```python
from build123d import *

# Parameters (mm, degrees)
BASE_FLANGE1_DEPTH       = 2.286
EDGE_FLANGE17_DEPTH      = 540.189115874
EDGE_FLANGE17_BEND_DEPTH = 539.451478538
EDGE_FLANGE18_DEPTH      = 357.000345524
EDGE_FLANGE18_BEND_DEPTH = 356.321109034
SKETCH197_R              = 12.065
CUT_EXTRUDE1_DEPTH       = 652.69497057


# Sheet-metal steps are written as plain solids
with BuildPart() as part:
    # Sketch1 → Base-Flange1 (new body)
    with BuildSketch(Plane(origin=(0, 0, 0), x_dir=(1, 0, 0), z_dir=(0, 1, 0))):
        Polygon((539.451478538, 356.320345524), (0, 356.320345524), (-0.737637336, 356.320345524), (0, 0), (539.451478538, 0), align=None)
    extrude(amount=-BASE_FLANGE1_DEPTH)

    # Edge-Flange17 section (across the edge) → Edge-Flange17 (add)
    with BuildSketch(Plane(origin=(-0.737637336, -2.286, -357.396945524), x_dir=(0, 0, 1), z_dir=(1, 0, 0))):
        with BuildLine():
            Line((-2.286, 0.7366), (-2.286, 16.15))
            Line((-2.286, 16.15), (0, 16.15))
            Line((0, 16.15), (0, 0.7366))
            ThreePointArc((0, 0.7366), (0.215745145, 0.215745145), (0.7366, 0))
            Line((0.7366, 0), (1.0766, 0))
            Line((1.0766, 0), (1.0766, -2.286))
            Line((1.0766, -2.286), (0.7366, -2.286))
            ThreePointArc((0.7366, -2.286), (-1.400700957, -1.400700957), (-2.286, 0.7366))
        make_face()
    extrude(amount=EDGE_FLANGE17_DEPTH)

    # Edge-Flange17 section 2 (across the edge) → Edge-Flange17 bend (add)
    with BuildSketch(Plane(origin=(539.451478538, -2.286, 1.0766), x_dir=(0, 0, -1), z_dir=(-1, 0, 0))):
        with BuildLine():
            Line((-2.286, 0.7366), (-2.286, 16.15))
            Line((-2.286, 16.15), (0, 16.15))
            Line((0, 16.15), (0, 0.7366))
            ThreePointArc((0, 0.7366), (0.215745145, 0.215745145), (0.7366, 0))
            Line((0.7366, 0), (1.0766, 0))
            Line((1.0766, 0), (1.0766, -2.286))
            Line((1.0766, -2.286), (0.7366, -2.286))
            ThreePointArc((0.7366, -2.286), (-1.400700957, -1.400700957), (-2.286, 0.7366))
        make_face()
    extrude(amount=EDGE_FLANGE17_BEND_DEPTH)

    # Edge-Flange18 section (across the edge) → Edge-Flange18 (add)
    with BuildSketch(Plane(origin=(540.848078538, -2.286, -356.660345524), x_dir=(-1, 0, 0), z_dir=(0, 0, 1))):
        with BuildLine():
            Line((-2.286, 0.7366), (-2.286, 16.15))
            Line((-2.286, 16.15), (0, 16.15))
            Line((0, 16.15), (0, 0.7366))
            ThreePointArc((0, 0.7366), (0.215745145, 0.215745145), (0.7366, 0))
            Line((0.7366, 0), (1.3966, 0))
            Line((1.3966, 0), (1.3966, -2.286))
            Line((1.3966, -2.286), (0.7366, -2.286))
            ThreePointArc((0.7366, -2.286), (-1.400700957, -1.400700957), (-2.286, 0.7366))
        make_face()
    extrude(amount=EDGE_FLANGE18_DEPTH)

    # Edge-Flange18 section 2 (across the edge) → Edge-Flange18 bend (add)
    with BuildSketch(Plane(origin=(-1.396597007, -2.286, 0.002891168), x_dir=(0.9999978572418866, -3.4914813388431337e-15, -0.0020701477327567633), z_dir=(-0.0020701477327567633, 0, -0.9999978572418866))):
        with BuildLine():
            Line((-2.286, 0.7366), (-2.286, 16.15))
            Line((-2.286, 16.15), (0, 16.15))
            Line((0, 16.15), (0, 0.7366))
            ThreePointArc((0, 0.7366), (0.215745145, 0.215745145), (0.7366, 0))
            Line((0.7366, 0), (1.3966, 0))
            Line((1.3966, 0), (1.3966, -2.286))
            Line((1.3966, -2.286), (0.7366, -2.286))
            ThreePointArc((0.7366, -2.286), (-1.400700957, -1.400700957), (-2.286, 0.7366))
        make_face()
    extrude(amount=EDGE_FLANGE18_BEND_DEPTH)

    # Sketch197 → Cut-Extrude1 (cut, through all)
    with BuildSketch(Plane(origin=(0, 0, 0), x_dir=(1, 0, 0), z_dir=(0, 1, 0))):
        with Locations(Location((486.180210266, 30.458714935, 0), (0, 0, 270))):
            Circle(SKETCH197_R)
        with Locations(Location((63.390735832, 29.575349793, 0), (0, 0, 270))):
            Circle(SKETCH197_R)
    extrude(amount=-CUT_EXTRUDE1_DEPTH, mode=Mode.SUBTRACT)


solid = part.part
```
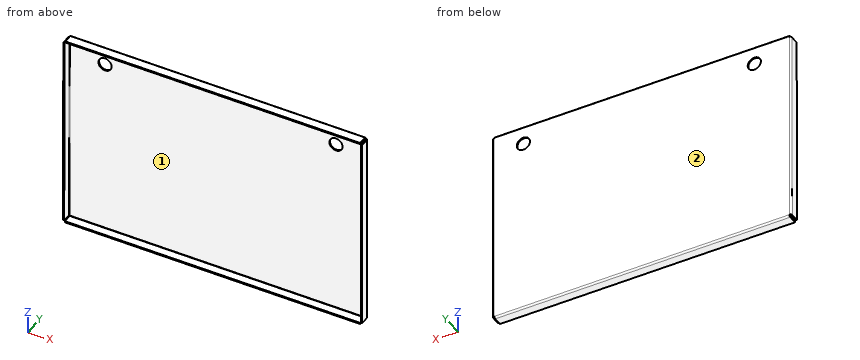
Here's how the part is built. I have some questions about the finished solid (model axes, mm). Face numbers are marked on the shaded views. Coordinates: 2 decimals unless noted, no trailing zeros. Order: outer loops, then holes, each group sorted by start corner. A loop starts at its lowest first (then second) coordinate and runs counter-clockwise, first axis right, second up. Notation, with made-up numbers: (65, 19) -> (123, 19) arc R28 cw to (123, 55) -> close; hole circle Ø4 at (22.5, 78). An arc over 180 degrees is marked (long way). Return JSON: item names as keys, results as strings.
1) Thinking about a two-plate mould opening in Z: for the marked faces 1 and 2, which applies, +Z half, -Z half, draft (parallel to the pull), parting line (faces both ways), or undercut?
Conclusion:
{"face 1": "undercut", "face 2": "draft"}
2) If we section it at A-A on y = -6.5: List the corners of the cut face in (x, z) for me, plus the area to 3 significant figures.
Conclusion:
{"outline": "(-4.42, -356.31) -> (-2.13, -356.32) -> (-1.4, 0) -> (-3.68, 0.01) -> close; (-0.74, -359.68) -> (539.45, -359.68) -> (539.45, -357.4) -> (-0.74, -357.4) -> close; (0, 1.08) -> (539.45, 1.08) -> (539.45, 3.36) -> (0, 3.36) -> close; (540.85, -356.66) -> (543.13, -356.66) -> (543.13, 0.34) -> (540.85, 0.34) -> close", "area": "4,100 mm²"}
3) If we section it at B-B on x = 220: List the corners of the cut face in (y, z) for me, plus the area to 3 significant figures.
Conclusion:
{"outline": "(-18.44, -359.68) -> (-3.02, -359.68) arc R3.02 ccw to (0, -356.66) -> (0, 0.34) arc R3.02 ccw to (-3.02, 3.36) -> (-18.44, 3.36) -> (-18.44, 1.08) -> (-3.02, 1.08) arc R0.74 cw to (-2.29, 0.34) -> (-2.29, -356.66) arc R0.74 cw to (-3.02, -357.4) -> (-18.44, -357.4) -> close", "area": "900 mm²"}
4) I'm going to push flat-ended pins straight in: P1, Ø1.5, axis at x = 201, z = -268, coming from the -Y side; P2, Ø3.5, axis at y = -5.5, z = 2.5, coming from the +X side; P3, Ø4, axis at x = 541.5, y = -6.5, coming from the +Z side. Where does each tip first touch, or does it pass through?
Conclusion:
{"P1": "stops at y = -2.29", "P2": "stops at x = 539.45", "P3": "stops at z = 0.34"}
5) If I drill on probe 1 along Z at (x, y) = (97.5, -4.5); probe 2 along Y at (x, z) = (503.5, -142); probe 3 along X at (y, z) = (-16.5, -229), over which ranges is the centre line in solid material (lowest first)?
Conclusion:
{"probe 1": "z = -359.68 to -357.4, 1.08 to 3.36", "probe 2": "y = -2.29 to 0", "probe 3": "x = -4.16 to -1.87, 540.85 to 543.13"}
